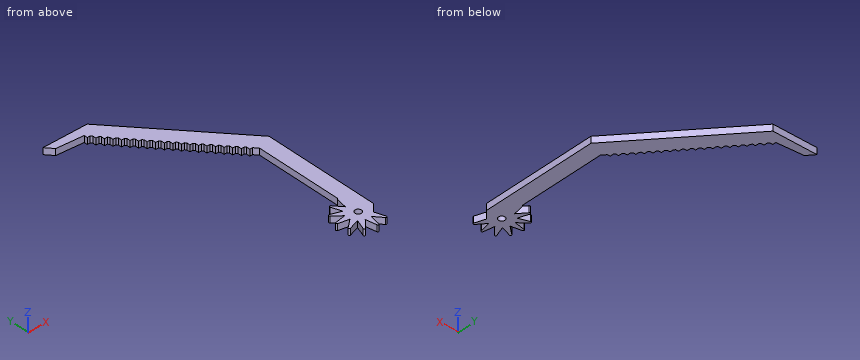
```python
from build123d import *

# Parameters (mm, degrees)
SKETCH2_R           = 8.75
BOSS_EXTRUDE1_DEPTH = 5
SKETCH2_3_R         = 2.5
CUT_EXTRUDE1_DEPTH  = 31
BOSS_EXTRUDE2_DEPTH = 5
CIRPATTERN2_COUNT   = 8
CIRPATTERN2_ANGLE   = 210
BOSS_EXTRUDE3_DEPTH = 5
BOSS_EXTRUDE4_START = -5
BOSS_EXTRUDE4_DEPTH = 5
CUT_EXTRUDE2_START  = -5
SKETCH7_R           = 2.5
CUT_EXTRUDE2_DEPTH  = 5
BOSS_EXTRUDE5_DEPTH = 5
LPATTERN1_COUNT     = 20
LPATTERN1_PITCH     = 5


with BuildPart() as part:
    # Sketch2 → Boss-Extrude1 (new body)
    with BuildSketch(Plane.XY):
        Circle(SKETCH2_R)
    extrude(amount=BOSS_EXTRUDE1_DEPTH)

    # Sketch2_3 → Cut-Extrude1 (cut)
    with BuildSketch(Plane.XY):
        Circle(SKETCH2_3_R)
    extrude(amount=CUT_EXTRUDE1_DEPTH, mode=Mode.SUBTRACT)

    # Sketch2_4 → Boss-Extrude2 (add)
    with BuildSketch(Plane.XY):
        with BuildLine():
            Line((0, 7.99133798), (-2.4, 7.99133798))
            Line((-2.4, 7.99133798), (-0.737233852, 16.887790594))
            ThreePointArc((-0.737233852, 16.887790594), (0, 17.5), (0.737233852, 16.887790594))
            Line((0.737233852, 16.887790594), (2.4, 7.99133798))
            Line((2.4, 7.99133798), (0, 7.99133798))
        make_face()
    boss_extrude2 = extrude(amount=BOSS_EXTRUDE2_DEPTH)

    # CirPattern2: Boss-Extrude2 ×8 about axis
    cirpattern2_axis = Axis((0, 0, 0), (0, 0, 1))
    for i in range(1, CIRPATTERN2_COUNT):
        add(boss_extrude2.rotate(cirpattern2_axis, i * CIRPATTERN2_ANGLE / (CIRPATTERN2_COUNT - 1)))



with BuildPart() as body_2:
    # Sketch5 → Boss-Extrude3 (new body)
    with BuildSketch(Plane.XY):
        Polygon((12, 85), (12, 90), (-58, 170), (-73, 170), (-92.6, 170), (-87.790588235, 164.4), (-66.790588235, 162.769863014), (0, 85), (0, 0), (12, 0), align=None)
    extrude(amount=BOSS_EXTRUDE3_DEPTH)


with BuildPart() as part_1:
    add(part.part)

    add(body_2.part)  # Boss-Extrude4 merges body 2
    # Sketch6 → Boss-Extrude4 (add)
    with BuildSketch(Plane.XY.offset(5).offset(BOSS_EXTRUDE4_START)):
        with BuildLine():
            ThreePointArc((8.75, 0), (8.175439475, -3.118443425), (6.527213853, -5.827347537))
            Line((6.527213853, -5.827347537), (12, 0))
            Line((12, 0), (8.75, 0))
        make_face()
    extrude(amount=BOSS_EXTRUDE4_DEPTH)

    # Sketch7 → Cut-Extrude2 (cut)
    with BuildSketch(Plane.XY.offset(5).offset(CUT_EXTRUDE2_START)):
        Circle(SKETCH7_R)
    extrude(amount=CUT_EXTRUDE2_DEPTH, mode=Mode.SUBTRACT)

    # Sketch8 → Boss-Extrude5 (add)
    with BuildSketch(Plane.XY.offset(5)):
        Polygon((-66.790588235, 162.769863014), (-66.790588235, 160.132718073), (-64.525746109, 160.132718073), align=None)
    boss_extrude5 = extrude(amount=-BOSS_EXTRUDE5_DEPTH)

    # LPattern1: Boss-Extrude5 ×20
    with Locations(*[Vector(0.651526069725241, -0.758626245570492, 0) * (i * LPATTERN1_PITCH) for i in range(1, LPATTERN1_COUNT)]):
        add(boss_extrude5)


solid = part_1.part
```
The listing builds one solid part. Answer for the finished solid, in the listing's coordinates (mm). Coordinates: 2 decimals unless noted, no trailing zeros. Loops run counter-clockwise (first coordinate to the right, second up) from the corner with the lowest first, then second, coordinate; pieces in that order, holes last. Notation, with made-up numbers: (86, 62.25) - (93, 62.25) arc R12 ccw to (93, 71.25) - close; hole circle Ø8 at (-24.75, 44.5). An arc over 180 degrees is marked (long way). Use a Markdown table: item, result. Add a question column.
1) The part is cut by section A-A, the plane y = 35. Give the vertices of the cut face in (x, z).
2) Find the intervals of material crossed by line 1 (X direction, y = 0, z = 3.2); line 2 (Y direction, x = -14, z = 2.2); line 3 (Y direction, x = -15.5, z = 2.4), in increasing order.
3) The part is cut by section B-B, the plane x = -82. Give the vertices of the cut face in (y, z), and give its area (3 significant figures).
4) Given pin 1 (1.1 mm diameter, centred on x = -59, z = 3.5, fed in from -Y); pin 2 (3 mm diameter, centred on y = 124, z = 3.5, fed in from -X); pin 3 (2 mm diameter, centred on x = -31, z = 1.5, fed in from -Y), each flat-ended and moving along its own axis, determine where each tip first touches the part or whether it passes through.
Here are the results:
| question | item | result |
|---|---|---|
| 1 | outline | (0, 0) - (12, 0) - (12, 5) - (0, 5) - close |
| 2 | line 1 | x = -17.5 to -2.5, 2.5 to 12 |
| 2 | line 2 | y = -8.99 to -6.95, -1.28 to 1.28, 6.95 to 8.99, 99.44 to 119.71 |
| 2 | line 3 | y = -1 to 1, 103.05 to 121.43 |
| 3 | outline | (163.95, 0) - (170, 0) - (170, 5) - (163.95, 5) - close |
| 3 | area | 30.2 mm^2 |
| 4 | pin 1 | stops at y = 152.55 |
| 4 | pin 2 | stops at x = -34.78 |
| 4 | pin 3 | stops at y = 118.41 |
